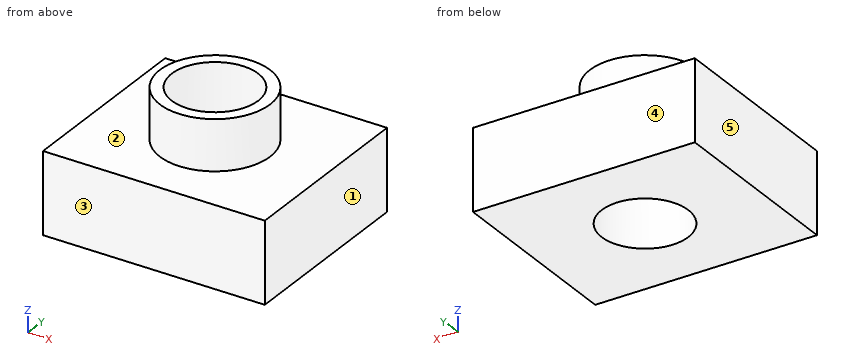
```python
from build123d import *

# Parameters (mm, degrees)
F0_W     = 152.4
F0_H     = 152.4
F1_DEPTH = 65.024
F2_R     = 34.6904695034
F3_DEPTH = 125.984
F4_R     = 44.1859582528
F4_R_2   = 34.6904695034
F5_DEPTH = 40.386
F6_DEPTH = 12.7
F7_DEPTH = 12.7


with BuildPart() as f1:
    # F0 (on Top) → F1 (new body)
    with BuildSketch(Plane.XY):
        Rectangle(F0_W, F0_H)
    extrude(amount=F1_DEPTH)

    # F2 (on face) → F3 (cut)
    with BuildSketch(Plane.XY.offset(65.024)):
        Circle(F2_R)
    extrude(amount=-F3_DEPTH, mode=Mode.SUBTRACT)

    # F4 (on face) → F5 (join)
    with BuildSketch(Plane.XY.offset(65.024)):
        Circle(F4_R)
        Circle(F4_R_2, mode=Mode.SUBTRACT)
    extrude(amount=F5_DEPTH)

    # F6 (add): a face of the model
    f6_faces = [f1.faces().sort_by_distance(p)[0] for p in [
        (76.2, 0, 32.512),
    ]]
    extrude(f6_faces, amount=F6_DEPTH)

    # F7 (add): a face of the model
    f7_faces = [f1.faces().sort_by_distance(p)[0] for p in [
        (-76.2, 0, 32.512),
    ]]
    extrude(f7_faces, amount=F7_DEPTH)


solid = f1.part
```
Input: part model. Units: mm. Frame: model coordinates. Face numbers are marked on the shaded views. A direction names the side the tool comes from. Coordinates: 2 decimals unless noted, no trailing zeros. Loops run counter-clockwise (first coordinate to the right, second up) from the corner with the lowest first, then second, coordinate; pieces in that order, holes last. Notation, with made-up numbers: M -32.5,-25 L -26.5,-25 A37 ccw -26.5,14 Z; hole C 36,63 d2. An arc over 180 degrees is marked long. Use a Markdown table: item, result. Add a question column.
1) Section C-C, the plane z = 12.5. Return the cut outline in (x, y), plus the area to 3 significant figures.
2) Draft query along Y for the marked faces 3, 4 and 5. Return one class per face: +Y half, -Y half, draft (parallel to the pull), parting line (faces both ways), or undercut.
3) Pin query (flat end, axial travel): P1, Ø6, axis at x = -27.5, z = 79, coming from the +Y side; P2, Ø4, axis at x = 48.5, y = -33.5, coming from the +Z side. Return the tip coordinate at first contact, or that it passes through.
4) Line query: L1, parallel to Y at x = 0, z = 95; L2, parallel to Y at x = 0, z = 33; L3, parallel to Z at x = -3.5, y = -56. Output: solid intervals per line, ascending. Write a range as from..to.
5) Set-up query: the marked faces 1 and 2. Return all of +Z, -Z, +X, -X, +Y, -Y with unobstructed straight access to the full face (end or side cutting, diameter ignored); none if empty.
6) Section A-A, the plane y = 0. Return the cut outline in (x, z).
7) Section D-D, the plane x = 39. Return the cut outline in (y, z), plus the area to 3 significant figures.
8) Section B-B, the plane x = 0. Return the cut outline in (y, z).
Answer below:
| question | item | result |
|---|---|---|
| 1 | outline | M -88.9,-76.2 L 88.9,-76.2 L 88.9,76.2 L -88.9,76.2 Z; hole C 0,0 d69.38 |
| 1 | area | 23,300 mm2 |
| 2 | face 3 | -Y half |
| 2 | face 4 | +Y half |
| 2 | face 5 | draft |
| 3 | P1 | y = 36.77 |
| 3 | P2 | z = 65.02 |
| 4 | L1 | -44.19..-34.69, 34.69..44.19 |
| 4 | L2 | -76.2..-34.69, 34.69..76.2 |
| 4 | L3 | 0..65.02 |
| 5 | face 1 | +Z, -Z, +X, +Y, -Y |
| 5 | face 2 | +Z |
| 6 | outline | M -88.9,0 L -34.69,0 L -34.69,105.41 L -44.19,105.41 L -44.19,65.02 L -88.9,65.02 Z; M 34.69,0 L 88.9,0 L 88.9,65.02 L 44.19,65.02 L 44.19,105.41 L 34.69,105.41 Z |
| 7 | outline | M -76.2,0 L 76.2,0 L 76.2,65.02 L 20.77,65.02 L 20.77,105.41 L -20.77,105.41 L -20.77,65.02 L -76.2,65.02 Z |
| 7 | area | 11,600 mm2 |
| 8 | outline | M -76.2,0 L -34.69,0 L -34.69,105.41 L -44.19,105.41 L -44.19,65.02 L -76.2,65.02 Z; M 34.69,0 L 76.2,0 L 76.2,65.02 L 44.19,65.02 L 44.19,105.41 L 34.69,105.41 Z |
